Verification items for the finished model (mm, model axes). Face numbers are marked on the shaded views. Round coordinates to 2 decimals unless told otherwise and drop trailing zeros. Write each loop counter-clockwise with the first axis right and the second up, starting at its lowest first coordinate (ties: lowest second). Pieces come first, ordered by that corner, then holes. Notation, with made-up numbers: M 28,-5.75 L 65,-5.75 A14 cw 65,3.25 Z; hole C 89.5,-31 d10. An arc over 180 degrees is marked long. One line per item, written item: value. Start each with the question number.
Item 1: Section check D-D, the plane z = -1.75. Record the cut outline in (x, y).
Item 2: Thickness scan on probe 1 along Y at (x, z) = (-7, -0.5); probe 2 along X at (y, z) = (7, 2); probe 3 along X at (y, z) = (6.25, -3). Record the ranges inside material, lowest first. Write a range as from..to.
Item 3: Section check C-C, the plane y = 9.25. Record the cut outline in (x, z).
Item 4: Section check B-B, the plane y = 13. Record the cut outline in (x, z).
Item 5: Gauge pin test, flat ends, axial feed: pin 1 (1 mm diameter, centred on x = 2, z = -1.5, fed in from -Y); pin 2 (3.5 mm diameter, centred on x = 6, y = 4.5, fed in from +Z); pin 3 (5 mm diameter, centred on y = 13, z = 4.5, fed in from -X). Record the tip position at first contact, or that the pin passes through.
Item 6: Draft check along X on the marked faces 1, 2, 3 and 4. Enter one of: +X half, -X half, draft (parallel to the pull), parting line (faces both ways), or undercut.
Item 7: Section check A-A, the plane z = -6.25. Record the cut outline in (x, y).
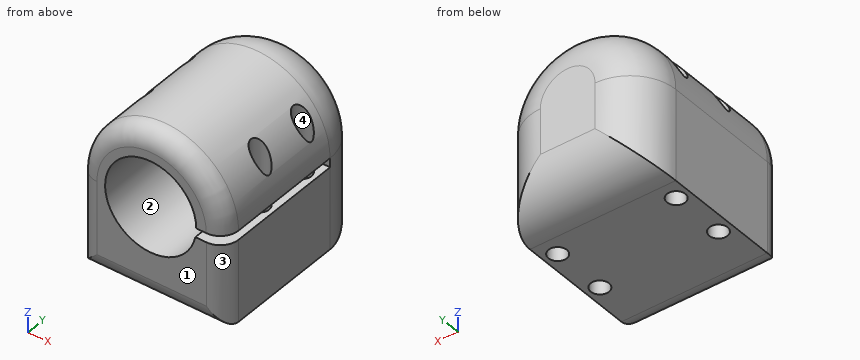
from build123d import *

# Parameters (mm, degrees)
BOSS_EXTRU_1_DEPTH           = 15
ESQUISSE3_R                  = 5
BOSS_EXTRU_3_DEPTH           = 5
ENL_V_MAT_EXTRU_2_REACH      = 30.071
ESQUISSE4_R                  = 1
ENL_V_MAT_EXTRU_3_REACH      = 29.495
ENL_V_MAT_EXTRU_3_END_RADIUS = 5
ESQUISSE5_W                  = 1
ESQUISSE5_H                  = 15
CONG_3_START                 = -10
CONG_3_DEPTH                 = 18
CONG_3_START_2               = -9
CONG_3_2_DEPTH               = 18
CONG_3_3_ANGLE               = 180
CONG_5_R                     = 2


with BuildPart() as part:
    # Esquisse1 → Boss.-Extru.1 (new body)
    with BuildSketch(Plane(origin=(0, 0, 0), x_dir=(1, 0, 0), z_dir=(0, 1, 0))):
        with BuildLine():
            ThreePointArc((-8, 0), (0, 8), (8, 0))
            Line((8, 0), (8, 10))
            Line((8, 10), (-8, 10))
            Line((-8, 10), (-8, 0))
        make_face()
        with BuildLine():
            ThreePointArc((-8, 0), (0, -8), (8, 0))
            Line((8, 0), (4.902542424, 0))
            ThreePointArc((4.902542424, 0), (-0.097457576, -5), (-5.097457576, 0))
            Line((-5.097457576, 0), (-8, 0))
        make_face()
        with BuildLine():
            Line((4.902542424, 0), (8, 0))
            ThreePointArc((8, 0), (0, 8), (-8, 0))
            Line((-8, 0), (-5.097457576, 0))
            ThreePointArc((-5.097457576, 0), (-0.097457576, 5), (4.902542424, 0))
        make_face()
    extrude(amount=BOSS_EXTRU_1_DEPTH)

    # Esquisse3 → Boss.-Extru.3 (add)
    # profile 1 of 3: a face of its own
    with BuildSketch(Plane(origin=(0, 15, 0), x_dir=(1, 0, 0), z_dir=(0, 1, 0))):
        with BuildLine():
            ThreePointArc((8, 0), (0, 8), (-8, 0))
            ThreePointArc((-8, 0), (0, -8), (8, 0))
        make_face()
        with Locations(Location((-0.097457576, 0, 0), (0, 0, 270))):
            Circle(ESQUISSE3_R, mode=Mode.SUBTRACT)
    # profile 2 of 3: a face of its own
    with BuildSketch(Plane(origin=(0, 15, 0), x_dir=(1, 0, 0), z_dir=(0, 1, 0))):
        with Locations(Location((-0.097457576, 0, 0), (0, 0, 270))):
            Circle(ESQUISSE3_R)
    # profile 3 of 3: a face of its own
    with BuildSketch(Plane(origin=(0, 15, 0), x_dir=(1, 0, 0), z_dir=(0, 1, 0))):
        with BuildLine():
            Line((-8, 10), (-8, 0))
            ThreePointArc((-8, 0), (0, 8), (8, 0))
            Line((8, 0), (8, 10))
            Line((8, 10), (-8, 10))
        make_face()
    extrude(amount=BOSS_EXTRU_3_DEPTH)

    # Esquisse4 → Enlèv. mat.-Extru.2 (cut, up to next)
    with BuildSketch(Plane(origin=(0, 0, -10), x_dir=(-1, 0, 0), z_dir=(0, 0, -1)), mode=Mode.PRIVATE) as enl_v_mat_extru_2_sk1:
        with Locations((-6.5, 13)):
            Circle(ESQUISSE4_R)
    enl_v_mat_extru_2_tool1 = extrude(enl_v_mat_extru_2_sk1.sketch, amount=-ENL_V_MAT_EXTRU_2_REACH, mode=Mode.PRIVATE) & part.part
    # Esquisse4 → Enlèv. mat.-Extru.2 (cut, up to next)
    with BuildSketch(Plane(origin=(0, 0, -10), x_dir=(-1, 0, 0), z_dir=(0, 0, -1)), mode=Mode.PRIVATE) as enl_v_mat_extru_2_sk2:
        with Locations((6.5, 13)):
            Circle(ESQUISSE4_R)
    enl_v_mat_extru_2_tool2 = extrude(enl_v_mat_extru_2_sk2.sketch, amount=-ENL_V_MAT_EXTRU_2_REACH, mode=Mode.PRIVATE) & part.part
    # Esquisse4 → Enlèv. mat.-Extru.2 (cut, up to next)
    with BuildSketch(Plane(origin=(0, 0, -10), x_dir=(-1, 0, 0), z_dir=(0, 0, -1)), mode=Mode.PRIVATE) as enl_v_mat_extru_2_sk3:
        with Locations((6.5, 7)):
            Circle(ESQUISSE4_R)
    enl_v_mat_extru_2_tool3 = extrude(enl_v_mat_extru_2_sk3.sketch, amount=-ENL_V_MAT_EXTRU_2_REACH, mode=Mode.PRIVATE) & part.part
    # Esquisse4 → Enlèv. mat.-Extru.2 (cut, up to next)
    with BuildSketch(Plane(origin=(0, 0, -10), x_dir=(-1, 0, 0), z_dir=(0, 0, -1)), mode=Mode.PRIVATE) as enl_v_mat_extru_2_sk4:
        with Locations((-6.5, 7)):
            Circle(ESQUISSE4_R)
    enl_v_mat_extru_2_tool4 = extrude(enl_v_mat_extru_2_sk4.sketch, amount=-ENL_V_MAT_EXTRU_2_REACH, mode=Mode.PRIVATE) & part.part
    add(enl_v_mat_extru_2_tool1.solids().sort_by_distance((6.5, 13, -10))[0], mode=Mode.SUBTRACT)
    add(enl_v_mat_extru_2_tool2.solids().sort_by_distance((-6.5, 13, -10))[0], mode=Mode.SUBTRACT)
    add(enl_v_mat_extru_2_tool3.solids().sort_by_distance((-6.5, 7, -10))[0], mode=Mode.SUBTRACT)
    add(enl_v_mat_extru_2_tool4.solids().sort_by_distance((6.5, 7, -10))[0], mode=Mode.SUBTRACT)

    # Enlèv. mat.-Extru.3: up to this cylinder (the profile starts outside it)
    enl_v_mat_extru_3_end = Plane(origin=(-0.097457576, 7.5, 0), z_dir=(0, -1, 0)) * Cylinder(ENL_V_MAT_EXTRU_3_END_RADIUS, 69.99, mode=Mode.PRIVATE)
    # Esquisse5 → Enlèv. mat.-Extru.3 (cut, up to the surface)
    with BuildSketch(Plane(origin=(8, 0, 0), x_dir=(0, 0, -1), z_dir=(1, 0, 0)), mode=Mode.PRIVATE) as enl_v_mat_extru_3_sk1:
        with Locations((0.5, 7.5)):
            Rectangle(ESQUISSE5_W, ESQUISSE5_H)
    enl_v_mat_extru_3_tool1 = extrude(enl_v_mat_extru_3_sk1.sketch, amount=-ENL_V_MAT_EXTRU_3_REACH, mode=Mode.PRIVATE) - enl_v_mat_extru_3_end
    add(enl_v_mat_extru_3_tool1.solids().sort_by_distance((8, 7.5, -0.5))[0], mode=Mode.SUBTRACT)

    # Congé3: read off the stored shape, not the designer's step
    # Congé3 outline → Congé3 (cut)
    with BuildSketch(Plane.XY.offset(CONG_3_START)):
        with BuildLine():
            ThreePointArc((-8, 15), (-6.535533906, 18.535533906), (-3, 20))
            Line((-3, 20), (-8, 20))
            Line((-8, 20), (-8, 15))
        make_face()
        with BuildLine():
            ThreePointArc((3, 20), (6.535533906, 18.535533906), (8, 15))
            Line((8, 15), (8, 20))
            Line((8, 20), (3, 20))
        make_face()
    extrude(amount=CONG_3_DEPTH, mode=Mode.SUBTRACT)

    # Cong_3 2 outline → Cong_3 2 (cut)
    with BuildSketch(Plane.YZ.offset(CONG_3_START_2)):
        with BuildLine():
            ThreePointArc((20, -5), (18.535533906, -8.535533906), (15, -10))
            Line((15, -10), (20, -10))
            Line((20, -10), (20, -5))
        make_face()
    extrude(amount=CONG_3_2_DEPTH, mode=Mode.SUBTRACT)

    # Cong_3 3 outline → Cong_3 3 (revolve, cut)
    with BuildSketch(Plane(origin=(0, 0, 0), x_dir=(-1, 0, 0), z_dir=(0, 0, -1))):
        with BuildLine():
            ThreePointArc((3, 20), (6.535533906, 18.535533906), (8, 15))
            Line((8, 15), (8, 20))
            Line((8, 20), (3, 20))
        make_face()
    revolve(axis=Axis((0, 0, 0), (0, 1, 0)), revolution_arc=CONG_3_3_ANGLE, mode=Mode.SUBTRACT)

    # Congé5
    cong_5_edges = [part.edges().sort_by_distance(p)[0] for p in [
        (8, 0, -5.5),
        (0, 0, -10),
        (0, 0, 8),
        (-8, 0, -5),
    ]]
    fillet(cong_5_edges, radius=CONG_5_R)


solid = part.part
Response values:
1. outline: M -8,2 A2 ccw -6,0 L -4.78,0 L -4.78,15 L 4.59,15 L 4.59,0 L 6,0 A2 ccw 8,2 L 8,15 A5 ccw 3,20 L -3,20 A5 ccw -8,15 Z; hole C -6.5,7 d2; hole C -6.5,13 d2; hole C 6.5,7 d2; hole C 6.5,13 d2
2. probe 1: y = 0.27..6.13, 7.87..12.13, 13.87..18
2. probe 2: x = -7.75..-7.5, -5.5..-4.68, 4.49..5.5, 7.5..7.75
2. probe 3: x = -8..-7.16, -5.84..-4.1, 3.9..5.84, 7.16..8
3. outline: M -8,-10 L 8,-10 L 8,-1 L 4.8,-1 A5 cw long 4.9,0 L 8,0 A8 ccw -8,0 Z
4. outline: M -8,-10 L -7.5,-10 L -7.5,2.78 A8 ccw -8,0 Z; M -5.5,-10 L 5.5,-10 L 5.5,-1 L 4.8,-1 A5 cw long 4.9,0 L 5.5,0 L 5.5,5.81 A8 ccw -5.5,5.81 Z; M 7.5,-10 L 8,-10 L 8,-1 L 7.5,-1 Z; M 7.5,0 L 8,0 A8 ccw 7.5,2.78 Z
5. pin 1: stops at y = 15
5. pin 2: stops at z = 6.78
5. pin 3: stops at x = -7.75
6. face 1: draft
6. face 2: undercut
6. face 3: +X half
6. face 4: undercut
7. outline: M -8,2 A2 ccw -6,0 L 6,0 A2 ccw 8,2 L 8,15 A5 ccw 4.25,19.84 L -4.25,19.84 A5 ccw -8,15 Z; hole C -6.5,7 d2; hole C -6.5,13 d2; hole C 6.5,7 d2; hole C 6.5,13 d2
